Check sheet for the drawn part. Datum: minimum x, y, z corner. Units: mm. Round coordinates to 2 decimals unless told otherwise and drop trailing zeros. Write each loop counter-clockwise with the first axis right and the second up, starting at its lowest first coordinate (ties: lowest second). Pieces come first, ordered by that corner, then holes.
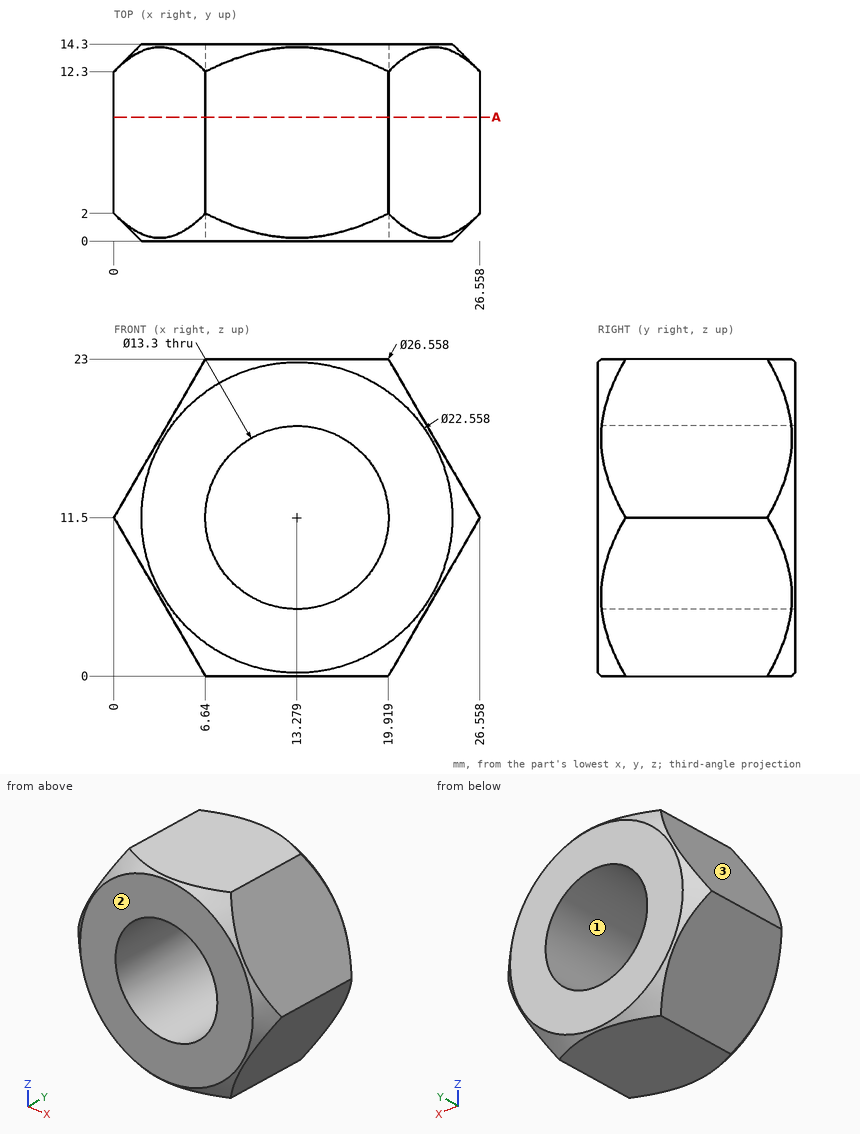
1. Scan lines: line 1 along Z through (x, y) = (13.5, 9.5); line 2 along X through (y, z) = (10.25, 12); line 3 along Z through (x, y) = (10.75, 10.5). Record each from-to range of solid material in increasing order.
2. Go/stop test with flat-tipped pins: pin 1 (8 mm diameter, centred on x = 15.5, z = 17.5, fed in from -Y); pin 2 (1 mm diameter, centred on x = 23.5, z = 17.5, fed in from -Y); pin 3 (5 mm diameter, centred on y = 9.5, z = 9.5, fed in from +X); pin 4 (10.5 mm diameter, centred on x = 13.28, z = 11.5, fed in from +Y). Record where each tip stops, or that it passes through.
3. Release check for a two-part mould opening along Z. For the marked faces 1, 2 and 3 record: released by +Z, released by -Z, zero draft, split by the parting line, or undercut.
4. Sectioned sample at A-A, the plane y = 9. Enter the section's corners in (x, z), plus the area to 3 significant figures.
Computed values:
1. line 1: z = 0 to 4.85, 18.15 to 23
1. line 2: x = 0.29 to 6.65, 19.91 to 26.27
1. line 3: z = 0 to 5.35, 17.65 to 23
2. pin 1: stops at y = 0
2. pin 2: stops at y = 0.07
2. pin 3: stops at x = 26.56
2. pin 4: passes through
3. face 1: undercut
3. face 2: zero draft
3. face 3: released by +Z
4. outline: (0, 11.5) - (6.64, 0) - (19.92, 0) - (26.56, 11.5) - (19.92, 23) - (6.64, 23) - close; hole circle Ø13.3 at (13.28, 11.5)
4. area: 319 mm2
